Verification items for this drawing (mm, ordinates from the low corner). Round coordinates to 2 decimals unless told otherwise and drop trailing zeros. Order: outer loops, then holes, each group sorted by start corner. A loop starts at its lowest first (then second) coordinate and runs counter-clockwise, first axis right, second up. Notation, with made-up numbers: (6.25, 38) -> (32.25, 38) arc R21 cw to (32.25, 56) -> close; hole circle Ø4 at (39.5, -40). An arc over 180 degrees is marked (long way). Answer in a Markdown table with one row per item.
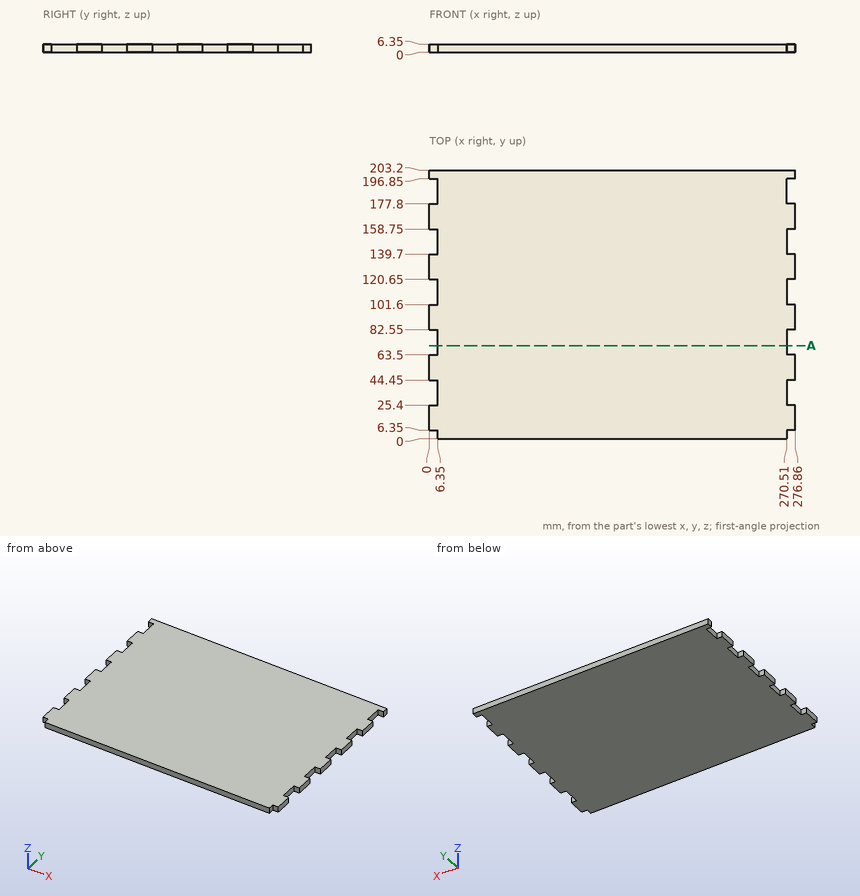
Item 1: Cross-section at A-A (y = 70.5). Record the boundary of the cut face in (x, z), and give its area (3 significant figures).
Result sheet:
| item | result |
|---|---|
| outline | (6.35, 0) -> (270.51, 0) -> (270.51, 6.35) -> (6.35, 6.35) -> close |
| area | 1,680 mm^2 |
Item 2: Scan line: line 1 (X direction, y = 76.5, z = 4.25). Record every from-to range of solid material in increasing order. Write a range as [from, to].
Result sheet:
| item | result |
|---|---|
| line 1 | x = [6.35, 270.51] |
Item 3: Depth check by flat-ended pin: P1, Ø3, axis at x = 2, z = 3.5, coming from the -Y side; P2, Ø1, axis at y = 32.5, z = 5, coming from the -X side; P3, Ø1.9, axis at y = 154, z = 2, coming from the +X side. Enter the tip coordinate at first touch or a pass-through.
Result sheet:
| item | result |
|---|---|
| P1 | stops at y = 6.35 |
| P2 | stops at x = 6.35 |
| P3 | stops at x = 270.51 |
